```python
from build123d import *

# Parameters (mm, degrees)
SKETCH1_R           = 25
SKETCH1_R_2         = 1.15
BOSS_EXTRUDE1_DEPTH = 6
SKETCH1_3_R         = 3.5
SKETCH1_3_R_2       = 1.15
BOSS_EXTRUDE2_DEPTH = 10
FILLET1_R           = 5
SKETCH2_W           = 0.5
SKETCH2_H           = 3


with BuildPart() as part:
    # Sketch1 → Boss-Extrude1 (new body)
    with BuildSketch(Plane(origin=(0, 0, 0), x_dir=(1, 0, 0), z_dir=(0, 1, 0))):
        with Locations(Location((0, 0, 0), (0, 0, 270))):
            Circle(SKETCH1_R)
        with Locations(Location((0, 0, 0), (0, 0, 270))):
            Circle(SKETCH1_R_2, mode=Mode.SUBTRACT)
    extrude(amount=BOSS_EXTRUDE1_DEPTH)

    # Sketch1<3> → Boss-Extrude2 (add)
    with BuildSketch(Plane(origin=(0, 0, 0), x_dir=(1, 0, 0), z_dir=(0, 1, 0))):
        with Locations(Location((0, 0, 0), (0, 0, 270))):
            Circle(SKETCH1_3_R)
        with Locations(Location((0, 0, 0), (0, 0, 270))):
            Circle(SKETCH1_3_R_2, mode=Mode.SUBTRACT)
    extrude(amount=BOSS_EXTRUDE2_DEPTH)

    # Fillet1
    # the kernel refuses this fillet: 5 mm, written as the material it adds along each edge
    with BuildSketch(Plane(origin=(0, 6, 0), x_dir=(0, 0, 1), z_dir=(1, 0, 0))) as fillet1_piece_1:
        with BuildLine():
            CenterArc((8.398979486, -5), FILLET1_R, 90, 78.463040967)
            Line((3.5, -4), (3.40202041, -3.98))
            ThreePointArc((3.40202041, -3.98), (3.4, -2), (3.4, 0))
            Line((3.4, 0), (3.5, 0.1))
            Line((3.5, 0.1), (8.398979486, 0.1))
            Line((8.398979486, 0.1), (8.398979486, 0))
        make_face()
    revolve(axis=Axis((0, 6, 0), (0, -1, 0)))

    # Sketch2 → Cut-Revolve1 (revolve, cut)
    with BuildSketch(Plane.XY, mode=Mode.PRIVATE) as cut_revolve1_sk:
        with Locations((24.75, 3)):
            Rectangle(SKETCH2_W, SKETCH2_H)
    revolve(cut_revolve1_sk.sketch.rotate(Axis((0, 6, 0), (0, -1, 0)), 90), axis=Axis((0, 6, 0), (0, -1, 0)), mode=Mode.SUBTRACT)


solid = part.part
```
The model under review builds one solid part; all positions refer to its coordinate system, in mm. A direction names the side the tool comes from. Coordinates: 2 decimals unless noted, no trailing zeros. Write each loop counter-clockwise with the first axis right and the second up, starting at its lowest first coordinate (ties: lowest second). Pieces come first, ordered by that corner, then holes. Notation, with made-up numbers: (62.5, 33) - (105.5, 33) arc R13 cw to (105.5, 50) - close; hole circle Ø10 at (55, -11). An arc over 180 degrees is marked (long way). Answer in a Markdown table with one row per item. Add a question column.
Q1. Clearance check with flat-ended pins moving along their axes: pin 1 (1.5 mm diameter, centred on y = 3, z = -8.5, fed in from +X); pin 2 (4 mm diameter, centred on x = 18.5, y = 8.5, fed in from -Z); pin 3 (1 mm diameter, centred on x = -13, z = 0, fed in from +Y); pin 4 (5 mm diameter, centred on y = 6.5, z = 15, fed in from +X). State where each tip first meets the part, or that it passes through.
Q2. Draft analysis for pull direction Y (two halves, no side actions). For faces 3 (the face through (0.345, 4.93, 1.097)), 4 (the face through (-11, 6, 0)), 5 (the face through (-7.36, 3.02, 23.37)), state which applies: +Y half, -Y half, draft (parallel to the pull), parting line (faces both ways), or undercut.
Q3. Consider section D-D on x = 22.5. Give the boundary of the cut face in (y, z), then the cut area to 3 significant figures.
Q4. For faces 1 (the face through (-5, 0, 0)), 2 (the face through (17, 1.5, -18)), list the 3-axis set-ups (+Z, -Z, +X, -X, +Y, -Y) from which the entire face can be reached by the end or side of a thin tool; tool diameter is ignored.
Q5. Consider section C-C on y = 3.5. Give the boundary of the cut face in (x, z), then the cut area to 3 significant figures.
Q6. To check wall thickness, follow line 1 along X through (y, z) = (3.25, 0); line 2 along X through (y, z) = (4.75, 0); line 3 along Y through (x, z) = (-20.5, -1). State the ranges of each line that lie inside material, in increasing order. Write a range as from..to.
Q7. Consider section A-A on z = 0. Give the boundary of the cut face in (x, y).
Q8. Consider section B-B on x = 0. Give the boundary of the cut face in (y, z).
Answers below:
| question | item | result |
|---|---|---|
| 1 | pin 1 | x = 23.24 |
| 1 | pin 2 | through |
| 1 | pin 3 | y = 6 |
| 1 | pin 4 | x = 21.62 |
| 2 | face 3 | draft |
| 2 | face 4 | +Y half |
| 2 | face 5 | undercut |
| 3 | outline | (0, -10.9) - (1.5, -10.9) - (1.5, -9.7) - (4.5, -9.7) - (4.5, -10.9) - (6, -10.9) - (6, 10.9) - (4.5, 10.9) - (4.5, 9.7) - (1.5, 9.7) - (1.5, 10.9) - (0, 10.9) - close |
| 3 | area | 124 mm² |
| 4 | face 1 | +Z, -Z, +X, -X, -Y |
| 4 | face 2 | none |
| 5 | outline | circle Ø49 at (0, 0); hole circle Ø2.3 at (0, 0) |
| 5 | area | 1,880 mm² |
| 6 | line 1 | -24.5..-1.15, 1.15..24.5 |
| 6 | line 2 | -25..-1.15, 1.15..25 |
| 6 | line 3 | 0..6 |
| 7 | outline | (-25, 0) - (-1.15, 0) - (-1.15, 10) - (-3.5, 10) arc R5 cw to (-8.4, 6) - (-25, 6) - (-25, 4.5) - (-24.5, 4.5) - (-24.5, 1.5) - (-25, 1.5) - close; (1.15, 0) - (25, 0) - (25, 1.5) - (24.5, 1.5) - (24.5, 4.5) - (25, 4.5) - (25, 6) - (8.4, 6) arc R5 cw to (3.5, 10) - (1.15, 10) - close |
| 8 | outline | (0, -25) - (1.5, -25) - (1.5, -24.5) - (4.5, -24.5) - (4.5, -25) - (6, -25) - (6, -8.4) arc R5 cw to (10, -3.5) - (10, -1.15) - (0, -1.15) - close; (0, 1.15) - (10, 1.15) - (10, 3.5) arc R5 cw to (6, 8.4) - (6, 25) - (4.5, 25) - (4.5, 24.5) - (1.5, 24.5) - (1.5, 25) - (0, 25) - close |
